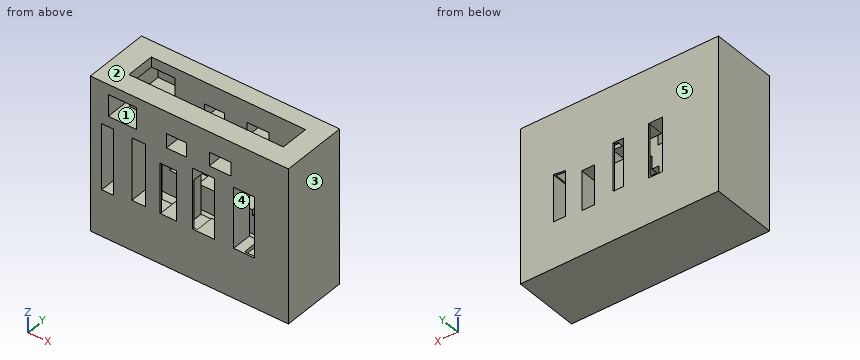
from build123d import *

# Parameters (mm, degrees)
F1_DEPTH = 60
F3_DEPTH = 10
F5_DEPTH = 25
F6_W     = 4.12122
F6_H     = 18.726911
F6_W_2   = 5.461499
F6_H_2   = 21.064218
F6_W_3   = 4.923844
F6_H_3   = 15.403733
F7_DEPTH = 25
F8_W     = 5.271911
F8_H     = 24.206938
F8_W_2   = 6.385386
F8_H_2   = 19.464375
F8_W_3   = 8.589027
F8_H_3   = 23.594679
F8_W_4   = 8.036524
F8_H_4   = 23.621964
F8_W_5   = 4.6295
F8_H_5   = 25.599981
F8_W_6   = 7.762552
F8_H_6   = 5.533628
F8_W_7   = 8.549511
F8_H_7   = 5.327355
F8_W_8   = 11.053609
F8_H_8   = 8.455139
F9_DEPTH = 25


with BuildPart() as f1:
    # F0 (on Top) → F1 (new body)
    with BuildSketch(Plane.XY):
        Polygon((-48.300002, -6.563763), (-48.300002, -17.85), (-48.300002, -25.725), (28.833047, -25.725), (28.833047, 0), (-48.300002, 0), align=None)
        Polygon((20.737499, -17.85), (-39.375003, -17.85), (-39.375003, -6.563763), (20.737499, -6.698824), align=None, mode=Mode.SUBTRACT)
    extrude(amount=F1_DEPTH)

    # F2 (on face) → F3 (join)
    with BuildSketch(Plane.XY):
        Polygon((-39.375003, -17.85), (20.737499, -17.85), (20.737499, -6.698824), (-39.375003, -6.563763), align=None)
    extrude(amount=F3_DEPTH)

    # F4 (on face) → F5 (cut)
    with BuildSketch(Plane(origin=(0, 0, 0), x_dir=(-1, 0, 0), z_dir=(0, 1, 0))):
        Polygon((-11.244134, 35.740558), (-16.007215, 36.322691), (-16.007215, 18.008349), (-11.244134, 18.008349), align=None)
    extrude(amount=-F5_DEPTH, mode=Mode.SUBTRACT)

    # F6 (on face) → F7 (cut)
    with BuildSketch(Plane(origin=(0, 0, 0), x_dir=(-1, 0, 0), z_dir=(0, 1, 0))):
        with Locations((9.246856, 28.394447)):
            Rectangle(F6_W, F6_H)
        with Locations((23.790132, 28.261853)):
            Rectangle(F6_W_2, F6_H_2)
        with Locations((-2.461922, 24.927176)):
            Rectangle(F6_W_3, F6_H_3)
    extrude(amount=-F7_DEPTH, mode=Mode.SUBTRACT)

    # F8 (on face) → F9 (cut)
    with BuildSketch(Plane.XZ.offset(25.725)):
        with Locations((-29.537439, 31.525831)):
            Rectangle(F8_W, F8_H)
        with Locations((-18.033631, 29.21811)):
            Rectangle(F8_W_2, F8_H_2)
        with Locations((-4.294513, 31.116555)):
            Rectangle(F8_W_3, F8_H_3)
        with Locations((11.522623, 31.159862)):
            Rectangle(F8_W_4, F8_H_4)
        with Locations((-41.608218, 30.823439)):
            Rectangle(F8_W_5, F8_H_5)
        with Locations((-14.784377, 48.786048)):
            Rectangle(F8_W_6, F8_H_6)
        with Locations((2.278485, 49.474218)):
            Rectangle(F8_W_7, F8_H_7)
        with Locations((-35.790155, 51.899684)):
            Rectangle(F8_W_8, F8_H_8)
    extrude(amount=-F9_DEPTH, mode=Mode.SUBTRACT)


solid = f1.part
The model under review builds one solid part; all positions refer to its coordinate system, in mm. Face numbers are marked on the shaded views. A direction names the side the tool comes from. Give positions to 0.01 mm unless a question says otherwise; leave off trailing zeros. Loops run counter-clockwise (first coordinate to the right, second up) from the corner with the lowest first, then second, coordinate; pieces in that order, holes last. Notation, with made-up numbers: (62.5, 67) -> (96.5, 67) arc R19 cw to (96.5, 79) -> close; hole circle Ø1 at (-7.75, -17.5). An arc over 180 degrees is marked (long way). Write each question's results on one line, items separated by ' | '.
1) Insertion check: pin 1 Ø1.8 at (x, y) = (-6, -4) entering from -Z; pin 2 Ø5.5 at (x, y) = (4.5, -14) entering from +Z. Each pin has a flat end and moves straight along its axis. Give the tip position at first contact, or say it passes through.
Conclusion:
pin 1: stops at z = 0 | pin 2: stops at z = 10
2) Take a section at A-A, the plane z = 48.5. Count the separate pieces of the cut face and the enclosed holes in it, plus the area to 3 significant figures.
Conclusion:
separate pieces: 3 | enclosed holes: 0 | area: 911 mm^2
3) Take a section at B-B, the plane x = -9.5. Give the boundary of the cut face in (y, z) (3 decimals), plus the area to 3 significant figures.
Conclusion:
outline: (-25.725, 0) -> (0, 0) -> (0, 19.031) -> (-6.631, 19.031) -> (-6.631, 10) -> (-17.85, 10) -> (-17.85, 19.031) -> (-25, 19.031) -> (-25, 37.758) -> (-17.85, 37.758) -> (-17.85, 60) -> (-25.725, 60) -> close; (-6.631, 37.758) -> (0, 37.758) -> (0, 60) -> (-6.631, 60) -> close | area: 724 mm^2
4) Tool access review of the marked faces 4 and 5: name each direction out of +Z, -Z, +X, -X, +Y, -Y from which nothing blocks a thin tool from reaching the whole face with its end or side.
Conclusion:
face 4: -Y | face 5: +Z, -Z, +X, -X, +Y
5) Take a section at C-C, the plane y = -9. Give the boundary of the cut face in (x, z) (1 decimal), plus the area to 3 significant figures.
Conclusion:
outline: (-48.3, 0) -> (28.8, 0) -> (28.8, 60) -> (20.7, 60) -> (20.7, 10) -> (-39.4, 10) -> (-39.4, 18) -> (-43.9, 18) -> (-43.9, 43.6) -> (-39.4, 43.6) -> (-39.4, 47.7) -> (-41.3, 47.7) -> (-41.3, 56.1) -> (-39.4, 56.1) -> (-39.4, 60) -> (-48.3, 60) -> close | area: 1,490 mm^2
6) For line 1 along X through (y, z) = (-1.5, 29.5); line 2 along X through (y, z) = (-23.5, 33); line 3 along Z through (x, y) = (-16.5, -6.5), list the stretches that pass through material, from the lowest coordinate up. Write a range as from..to.
Conclusion:
line 1: x = -48.3..-43.92, -39.29..-32.17, -26.9..-26.52, -14.84..-11.31, 4.92..7.5, 16.01..28.83 | line 2: x = -48.3..-43.92, -39.29..-32.17, -26.9..-26.52, -14.84..-11.31, 0..7.5, 16.01..28.83 | line 3: z = 0..19.49, 38.95..46.02, 51.55..60
7) Take a section at D-D, the plane x = -42.5. Give the boundary of the cut face in (y, z) (3 decimals), plus the area to 4 significant figures.
Conclusion:
outline: (-25.725, 0) -> (0, 0) -> (0, 60) -> (-25.725, 60) -> (-25.725, 43.623) -> (-0.725, 43.623) -> (-0.725, 18.023) -> (-25.725, 18.023) -> close | area: 903.5 mm^2
8) Draft analysis for pull direction X (two halves, no side actions). For the marked faces 1, 2 and 3, state which applies: pulls with the +X half, pulls with the -X half, needs draft (parallel to the pull), parting line crosses it, or undercut.
Conclusion:
face 1: undercut | face 2: needs draft | face 3: pulls with the +X half
